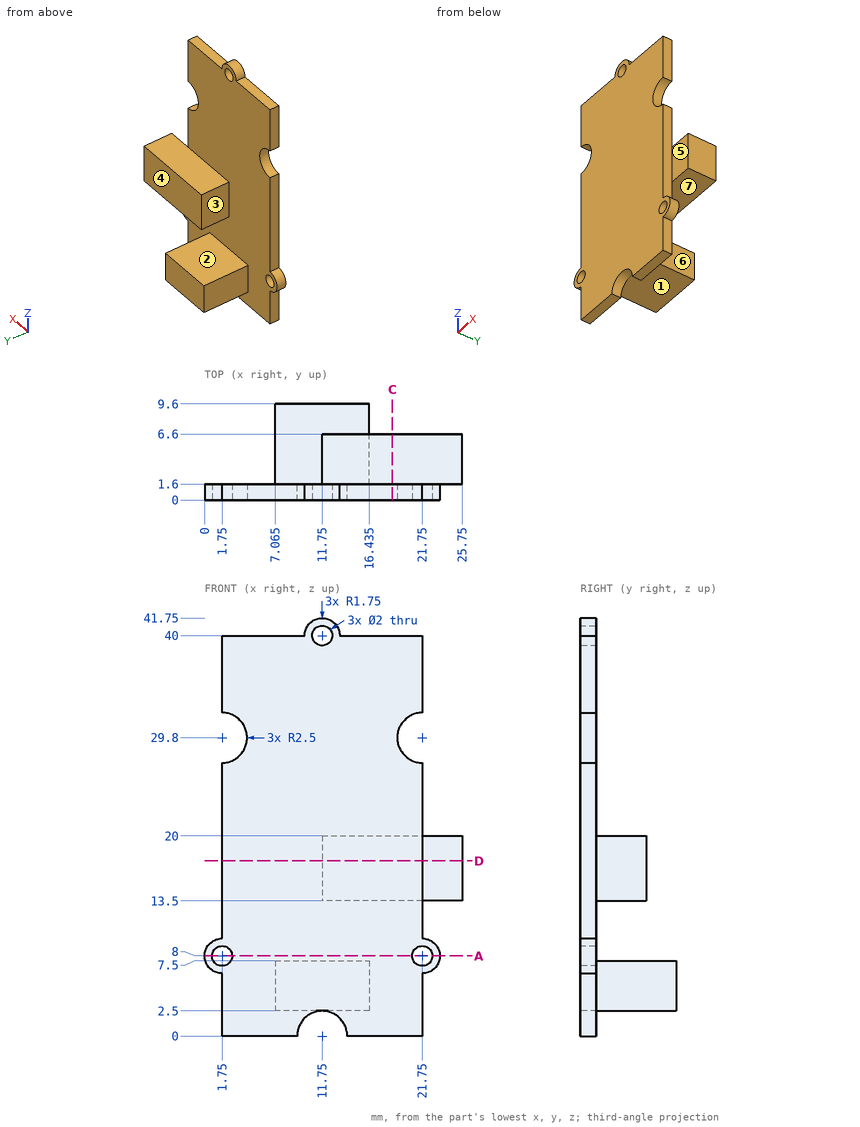
Could you check a few things on this drawing? It's one solid part, dimensions in mm from its lowest x, y, z. A direction names the side the tool comes from. Round coordinates to 2 decimals unless told otherwise and drop trailing zeros. Order: outer loops, then holes, each group sorted by start corner. A loop starts at its lowest first (then second) coordinate and runs counter-clockwise, first axis right, second up. Notation, with made-up numbers: M -25.5,-17 L 32.5,-17 A5 ccw 32.5,-10 Z; hole C -24.75,88.25 d9. An arc over 180 degrees is marked long. One line per question, with ' | ' between items.
1) We'd pull the mould along Z, two halves only. Please class the marked faces 1, 2 and 3: released by +Z, released by -Z, zero draft, split by the parting line, or undercut.
Checked values:
face 1: released by -Z | face 2: undercut | face 3: zero draft
2) Imagine slicing it at A-A, the plane z = 8. Write out the boundary of the cut face in (x, y), plus the area to 3 significant figures.
Checked values:
outline: M 0,0 L 0.75,0 L 0.75,1.6 L 0,1.6 Z; M 2.75,0 L 20.75,0 L 20.75,1.6 L 2.75,1.6 Z; M 22.75,0 L 23.5,0 L 23.5,1.6 L 22.75,1.6 Z | area: 31.2 mm²
3) Imagine slicing it at D-D, the plane z = 17.5. Write out the boundary of the cut face in (x, y), plus the area to 3 significant figures.
Checked values:
outline: M 1.75,0 L 21.75,0 L 21.75,1.6 L 25.75,1.6 L 25.75,6.6 L 11.75,6.6 L 11.75,1.6 L 1.75,1.6 Z | area: 102 mm²
4) I'm going to push flat-ended pins straight in: pin 1 Ø0.8 at (y, z) = (1, 16.5) entering from +X; pin 2 Ø4 at (x, y) = (22, 5) entering from -Z; pin 3 Ø12 at (x, z) = (14.5, 27.5) entering from +Y. Where does each tip first touch, or does it pass through?
Checked values:
pin 1: stops at x = 21.75 | pin 2: stops at z = 13.5 | pin 3: stops at y = 1.6
5) On a 3-axis mill with a long thin cutter (end or side, diameter ignored), from which of +Z, -Z, +X, -X, +Y, -Y can I reach the whole of each face in a straight line? I mean the marked faces 4, 5, 6 and 7. Say none if no direction works.
Checked values:
face 4: +Z, +X, -X, +Y | face 5: +Z, +X, -Y | face 6: -Z, +X, +Y | face 7: +X, -X, +Y
6) I need wall thicknesses on line 1 (X direction, y = 0.55, z = 8); line 2 (X direction, y = 4, z = 3.5) (1 decimal); line 3 (Y direction, x = 17, z = 26). Which ranges of each line are inside material? Lowest first, please.
Checked values:
line 1: x = 0 to 0.75, 2.75 to 20.75, 22.75 to 23.5 | line 2: x = 7.1 to 16.4 | line 3: y = 0 to 1.6
7) Imagine slicing it at C-C, the plane x = 18.75. Write out the boundary of the cut face in (y, z).
Checked values:
outline: M 0,0 L 1.6,0 L 1.6,13.5 L 6.6,13.5 L 6.6,20 L 1.6,20 L 1.6,40 L 0,40 Z
